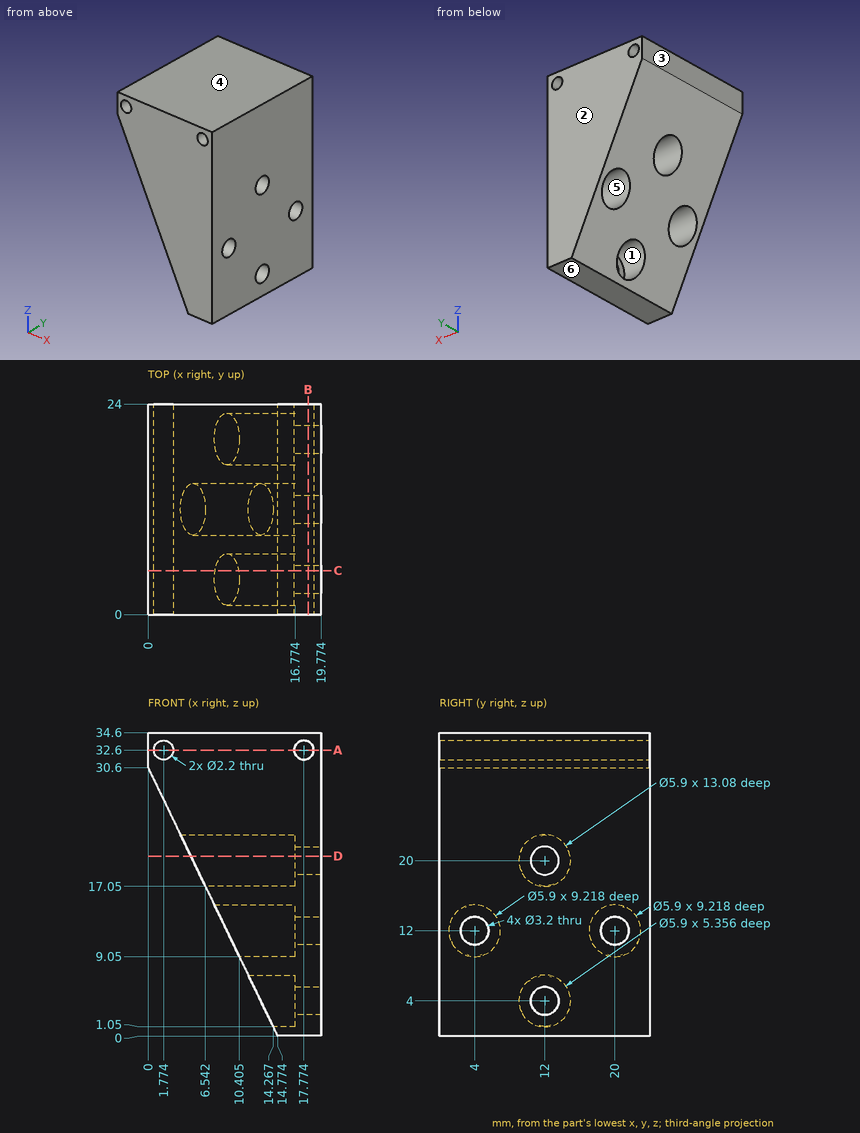
For this review, use the dimensioned drawing (mm, ordinates from the lowest corner) and the shaded views. A direction names the side the tool comes from. Coordinates: 2 decimals unless noted, no trailing zeros. Loops run counter-clockwise (first coordinate to the right, second up) from the corner with the lowest first, then second, coordinate; pieces in that order, holes last. Notation, with made-up numbers: (26, 65) - (31, 65) arc R27 cw to (31, 104) - close; hole circle Ø6 at (84, -2.5). An arc over 180 degrees is marked (long way). Use CSV: the item, a comma, the result in double quotes. Start each with the question number.
1) Consider section D-D on z = 20.5. Write out the cut boundary in (x, y) (1 decimal), then the cut area to 3 significant figures.
2) Consider section A-A on z = 32.6. Write out the cut boundary in (x, y) (1 decimal).
3) The part is to be moulded in two halves that separate along Z. For the marked faces 3, 4, 5 and 6, say which applies: +Z half, -Z half, draft (parallel to the pull), parting line (faces both ways), or undercut.
4) For pin 1 Ø1.8 at (y, z) = (12, 4) entering from -X; pin 2 Ø4 at (x, y) = (6.5, 6.5) entering from -Z; pin 3 Ø3 at (y, z) = (20.5, 12) entering from -X; pin 4 Ø6 at (y, z) = (20, 23) entering from -X, all flat-tipped, find the tip position at first contact; note any pin that passes through.
5) Consider section B-B on x = 18.25. Write out the cut boundary in (y, z).
6) Consider section C-C on y = 5. Give the number of separate pieces and of enclosed holes in the cut face, then the cut area to 3 significant figures.
7) Tool access review of the marked faces 1 and 2: name each direction out of +Z, -Z, +X, -X, +Y, -Y from which nothing blocks a thin tool from reaching the whole face with its end or side.
8) Wall thickness on L1, parallel to Y at x = 13.5, z = 12; L2, parallel to Z at x = 18.15, y = 20 (1 decimal); L3, parallel to Y at x = 18.5, z = 20: over which ranges is each line inside the solid? List them lowest first. Write a range as from..to.
Geometry says:
1,outline,"(4.9, 0) - (19.8, 0) - (19.8, 10.5) - (16.8, 10.5) - (16.8, 9.1) - (4.9, 9.1) - close; (4.9, 14.9) - (16.8, 14.9) - (16.8, 13.5) - (19.8, 13.5) - (19.8, 24) - (4.9, 24) - close"
1,area,"279 mm^2"
2,outline,"(0, 0) - (0.7, 0) - (0.7, 24) - (0, 24) - close; (2.9, 0) - (16.7, 0) - (16.7, 24) - (2.9, 24) - close; (18.9, 0) - (19.8, 0) - (19.8, 24) - (18.9, 24) - close"
3,face 3,"draft"
3,face 4,"+Z half"
3,face 5,"undercut"
3,face 6,"-Z half"
4,pin 1,"through"
4,pin 2,"z = 13.03"
4,pin 3,"x = 16.77"
4,pin 4,"x = 2.22"
5,outline,"(0, 0) - (24, 0) - (24, 31.61) - (0, 31.61) - close; (0, 33.59) - (24, 33.59) - (24, 34.6) - (0, 34.6) - close; hole circle Ø3.2 at (4, 12); hole circle Ø3.2 at (12, 4); hole circle Ø3.2 at (12, 20); hole circle Ø3.2 at (20, 12)"
6,separate pieces,"2"
6,enclosed holes,"2"
6,area,"400 mm^2"
7,face 1,"-X"
7,face 2,"+Z, -Z, +X, -X, +Y"
8,L1,"0..1.05, 6.95..17.05, 22.95..24"
8,L2,"0..10.4, 13.6..31.6, 33.6..34.6"
8,L3,"0..10.4, 13.6..24"
